```python
from build123d import *

# Parameters (mm, degrees)
F0_W        = 126.111
F0_H        = 164.9984
F0_W_2      = 121.031
F0_H_2      = 159.9184
F1_DEPTH    = 25.4
F1_FACE_W   = 126.111
F1_FACE_H   = 164.9984
F1_FACE_W_2 = 121.031
F1_FACE_H_2 = 159.9184
F2_DEPTH    = 2.54
F4_DEPTH    = 164.9984
F5_W        = 98.6028
F5_H        = 127.0508
F6_DEPTH    = 25.4


with BuildPart() as f1:
    # F0 (on Right) → F1 (new body)
    with BuildSketch(Plane.YZ):
        with Locations((27.1188945978, -12.7647293852)):
            Rectangle(F0_W, F0_H)
        with Locations((27.1188945978, -12.7647293852)):
            Rectangle(F0_W_2, F0_H_2, mode=Mode.SUBTRACT)
    extrude(amount=F1_DEPTH)

    # F1_face (on face) + F0 (on Right) → F2 (join)
    with BuildSketch(Plane(origin=(0, 27.1188945978, -12.7647293852), x_dir=(0, 1, 0), z_dir=(-1, 0, 0))):
        Rectangle(F1_FACE_W, F1_FACE_H)
        Rectangle(F1_FACE_W_2, F1_FACE_H_2, mode=Mode.SUBTRACT)
    with BuildSketch(Plane.YZ):
        with Locations((27.1188945978, -12.7647293852)):
            Rectangle(F0_W, F0_H)
        with Locations((27.1188945978, -12.7647293852)):
            Rectangle(F0_W_2, F0_H_2, mode=Mode.SUBTRACT)
        with Locations((27.1188945978, -12.7647293852)):
            Rectangle(F0_W_2, F0_H_2)
    extrude(amount=F2_DEPTH, dir=(-1, 0, 0))

    # F3 (on face) → F4 (join)
    with BuildSketch(Plane.XY.offset(69.7344706148)):
        Polygon((-2.54, 87.6343945978), (-2.54, 90.1743945978), (-18.288, 90.1743945978), (-18.288, 80.0143945978), (-15.748, 80.0143945978), (-15.748, 87.6343945978), align=None)
        Polygon((-2.54, -35.9366054022), (-2.54, -33.4024998063), (-15.748, -33.4024998063), (-15.748, -25.7766054022), (-18.288, -25.7766054022), (-18.288, -35.9366054022), align=None)
    extrude(amount=-F4_DEPTH)

    # F5 (on face) → F6 (cut)
    with BuildSketch(Plane.YZ):
        with Locations((27.1188945978, -12.6885293852)):
            Rectangle(F5_W, F5_H)
    extrude(amount=-F6_DEPTH, mode=Mode.SUBTRACT)


solid = f1.part
```
For this review, take the finished solid that the model builds, in its own axes (mm). A direction names the side the tool comes from. Coordinates: 2 decimals unless noted, no trailing zeros. Order: outer loops, then holes, each group sorted by start corner. A loop starts at its lowest first (then second) coordinate and runs counter-clockwise, first axis right, second up. Notation, with made-up numbers: (-27.5, 3.5) - (21.5, 3.5) arc R7 cw to (21.5, 7.5) - close; hole circle Ø1 at (24.25, -36). An arc over 180 degrees is marked (long way). Answer as a JSON object with one key per item and string values. Group by question number.
1. We need section C-C on x = -12. State the section outline as (y, z) points, then the cut area to 3 significant figures.
2. The part is to be moulded in two halves that separate along Y. For faces 1 (the flat face through (-9, 87.634, -12)), 2 (the flat face through (4, 90.174, -12)), 3 (the flat face through (4, -35.937, -12)), 4 (the flat face through (8, 28, 69.734)), say which applies: pulls with the +Y half, pulls with the -Y half, needs draft (parallel to the pull), parting line crosses it, or undercut.
3. We need section A-A on y = 45.5. State the section outline as (x, z) points, then the cut area to 3 significant figures.
4. Clearance check with flat-ended pins moving along their axes: P1, Ø1.5, axis at x = -4.5, y = 40, coming from the +Z side; P2, Ø2.5, axis at y = 82.5, z = -2, coming from the +X side. State where each tip first meets the part, or that it passes through.
5. For probe 1 along Y at (x, z) = (23.5, -21); probe 2 along Z at (x, y) = (7, 26.5); probe 3 along X at (y, z) = (-14.5, -88), list the stretches that pass through material, from the lowest coordinate up.
6. We need section B-B on z = -25.5. State the section outline as (x, y) points, then the cut area to 3 significant figures.
7. For faces 5 (the flat face through (13, 26, -92.724)), 6 (the flat face through (-18.288, 85, -12)), 7 (the flat face through (-9, -33.402, -12)), list the 3-axis set-ups (+Z, -Z, +X, -X, +Y, -Y) from which the entire face can be reached by the end or side of a thin tool; tool diameter is ignored.
8. We need section D-D on x = 11. State the section outline as (y, z) points, then the cut area to 3 significant figures.
Final values:
{
 "1": {"outline": "(-35.94, -95.26) - (-33.4, -95.26) - (-33.4, 69.73) - (-35.94, 69.73) - close; (87.63, -95.26) - (90.17, -95.26) - (90.17, 69.73) - (87.63, 69.73) - close", "area": "837 mm²"},
 "2": {"face 1": "undercut", "face 2": "pulls with the +Y half", "face 3": "pulls with the -Y half", "face 4": "needs draft"},
 "3": {"outline": "(-2.54, -95.26) - (25.4, -95.26) - (25.4, -92.72) - (0, -92.72) - (0, -76.21) - (-2.54, -76.21) - close; (-2.54, 50.84) - (0, 50.84) - (0, 67.19) - (25.4, 67.19) - (25.4, 69.73) - (-2.54, 69.73) - close", "area": "225 mm²"},
 "4": {"P1": "through", "P2": "x = 0"},
 "5": {"probe 1": "-35.94 to -33.4, 87.63 to 90.17", "probe 2": "-95.26 to -92.72, 67.19 to 69.73", "probe 3": "-2.54 to 0"},
 "6": {"outline": "(-18.29, -35.94) - (25.4, -35.94) - (25.4, -33.4) - (0, -33.4) - (0, -22.18) - (-2.54, -22.18) - (-2.54, -33.4) - (-15.75, -33.4) - (-15.75, -25.78) - (-18.29, -25.78) - close; (-18.29, 80.01) - (-15.75, 80.01) - (-15.75, 87.63) - (-2.54, 87.63) - (-2.54, 76.42) - (0, 76.42) - (0, 87.63) - (25.4, 87.63) - (25.4, 90.17) - (-18.29, 90.17) - close", "area": "318 mm²"},
 "7": {"face 5": "+X", "face 6": "+Z, -Z, -X, +Y, -Y", "face 7": "+Z, -Z"},
 "8": {"outline": "(-35.94, -95.26) - (90.17, -95.26) - (90.17, 69.73) - (-35.94, 69.73) - close; hole (-33.4, -92.72) - (87.63, -92.72) - (87.63, 67.19) - (-33.4, 67.19) - close", "area": "1,450 mm²"}
}
